The listing builds one solid part. Answer for the finished solid, in the listing's coordinates (mm). Face numbers are marked on the shaded views. A direction names the side the tool comes from. Give positions to 0.01 mm unless a question says otherwise; leave off trailing zeros. Loops run counter-clockwise (first coordinate to the right, second up) from the corner with the lowest first, then second, coordinate; pieces in that order, holes last. Notation, with made-up numbers: M 71,36 L 77,36 A29 ccw 77,73 Z; hole C -2,58.25 d5. An arc over 180 degrees is marked long. Return JSON: item names as keys, results as strings.
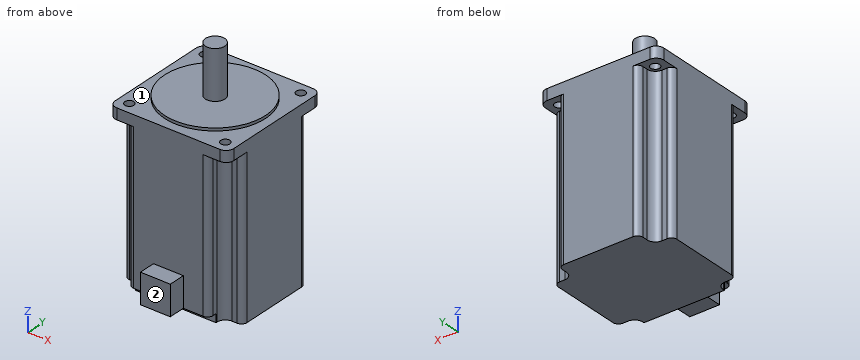
from build123d import *

# Parameters (mm, degrees)
SZKIC7_W                    = 21.6
SZKIC7_H                    = 21.6
DODANIE_WYCI_GNI_CIE5_DEPTH = 12
SZKIC8_W                    = 85.8
SZKIC8_H                    = 115
DODANIE_WYCI_GNI_CIE6_DEPTH = 85.8
SZKIC9_W                    = 85.8
SZKIC9_H                    = 78.988293657
DODANIE_WYCI_GNI_CIE7_DEPTH = 7
SZKIC10_W                   = 113
SZKIC10_H                   = 16.646355961
WYTNIJ_WYCI_GNI_CIE3_DEPTH  = 13.8
SZKIC11_W                   = 13.8
SZKIC11_H                   = 113
WYTNIJ_WYCI_GNI_CIE4_DEPTH  = 13.8
SZKIC12_W                   = 113
SZKIC12_H                   = 13.8
WYTNIJ_WYCI_GNI_CIE5_DEPTH  = 13.8
SZKIC13_W                   = 13.8
SZKIC13_H                   = 113
WYTNIJ_WYCI_GNI_CIE6_DEPTH  = 13.8
SZKIC14_R                   = 36.51
DODANIE_WYCI_GNI_CIE8_DEPTH = 2
OTW_R_POD_RUB_M121_D        = 14.05
OTW_R_POD_RUB_M121_DEPTH    = 2
SZKIC17_W                   = 7
SZKIC17_H                   = 37
OTW_R_6_6_6_6_1_D           = 6.6
OTW_R_6_6_6_6_1_DEPTH       = 45
ZAOKR_GLENIE1_R             = 4.000000016
ZAOKR_GLENIE2_R             = 5.6
ZAOKR_GLENIE3_R             = 5.99999999


with BuildPart() as part:
    # Szkic7 → Dodanie-wyciągnięcie5 (new body)
    with BuildSketch(Plane(origin=(0, -55, 0), x_dir=(-1, 0, 0), z_dir=(0, 1, 0))):
        with Locations((0, -104.2)):
            Rectangle(SZKIC7_W, SZKIC7_H)
    extrude(amount=DODANIE_WYCI_GNI_CIE5_DEPTH)

    # Szkic8 → Dodanie-wyciągnięcie6 (add)
    with BuildSketch(Plane(origin=(0, -43, 0), x_dir=(-1, 0, 0), z_dir=(0, 1, 0))):
        with Locations((0, -57.5)):
            Rectangle(SZKIC8_W, SZKIC8_H)
    extrude(amount=DODANIE_WYCI_GNI_CIE6_DEPTH)

    # Szkic9 → Dodanie-wyciągnięcie7 (add)
    with BuildSketch(Plane(origin=(0, 0, -121), x_dir=(-1, 0, 0), z_dir=(0, 0, -1))):
        with Locations((0, 3.305853172)):
            Rectangle(SZKIC9_W, SZKIC9_H)
    extrude(amount=-DODANIE_WYCI_GNI_CIE7_DEPTH)

    # Szkic10 → Wytnij-wyciągnięcie3 (cut)
    with BuildSketch(Plane.ZY.offset(42.9)):
        with Locations((-64.5, -37.423177981)):
            Rectangle(SZKIC10_W, SZKIC10_H)
    extrude(amount=-WYTNIJ_WYCI_GNI_CIE3_DEPTH, mode=Mode.SUBTRACT)

    # Szkic11 → Wytnij-wyciągnięcie4 (cut)
    with BuildSketch(Plane.XZ.offset(43)):
        with Locations((36, -64.5)):
            Rectangle(SZKIC11_W, SZKIC11_H)
    extrude(amount=-WYTNIJ_WYCI_GNI_CIE4_DEPTH, mode=Mode.SUBTRACT)

    # Szkic12 → Wytnij-wyciągnięcie5 (cut)
    with BuildSketch(Plane(origin=(42.9, 0, 0), x_dir=(0, 0, -1), z_dir=(1, 0, 0))):
        with Locations((64.5, 36)):
            Rectangle(SZKIC12_W, SZKIC12_H)
    extrude(amount=-WYTNIJ_WYCI_GNI_CIE5_DEPTH, mode=Mode.SUBTRACT)

    # Szkic13 → Wytnij-wyciągnięcie6 (cut)
    with BuildSketch(Plane(origin=(0, 42.8, 0), x_dir=(-1, 0, 0), z_dir=(0, 1, 0))):
        with Locations((36, -64.5)):
            Rectangle(SZKIC13_W, SZKIC13_H)
    extrude(amount=-WYTNIJ_WYCI_GNI_CIE6_DEPTH, mode=Mode.SUBTRACT)

    # Szkic14 → Dodanie-wyciągnięcie8 (add)
    with BuildSketch(Plane.XY):
        with Locations(Location((0, 0, 0), (0, 0, 90))):
            Circle(SZKIC14_R)
    extrude(amount=DODANIE_WYCI_GNI_CIE8_DEPTH)

    # Otwór pod śrubę M121
    with Locations(Plane.XY.offset(2)):
        with Locations((0, 0)):
            Hole(OTW_R_POD_RUB_M121_D / 2, depth=OTW_R_POD_RUB_M121_DEPTH)

    # Szkic17 → Obrót1 (revolve)
    with BuildSketch(Plane(origin=(0, 0, 0), x_dir=(1, 0, 0), z_dir=(0, 1, 0))):
        with Locations((3.5, -18.5)):
            Rectangle(SZKIC17_W, SZKIC17_H)
    revolve(axis=Axis((0, 0, 0), (0, 0, 1)))

    # Otwór Ø6.6 (6.6)1
    with Locations(Plane(origin=(0, 0, -8), x_dir=(-1, 0, 0), z_dir=(0, 0, -1))):
        with Locations((34.718942956, -34.718942956), (-34.718942956, -34.718942956), (-34.718942956, 34.718942956), (34.718942956, 34.718942956)):
            Hole(OTW_R_6_6_6_6_1_D / 2, depth=OTW_R_6_6_6_6_1_DEPTH)

    # Zaokrąglenie1
    zaokr_glenie1_edges = [part.edges().sort_by_distance(p)[0] for p in [
        (-42.9, 29, -64.5),
        (-29.1, 42.8, -64.5),
        (-29.1, -43, -61.5),
        (-42.9, -29.1, -64.5),
        (29.1, -43, -61.5),
        (42.9, -29.2, -64.5),
        (42.9, 29.1, -64.5),
        (29.1, 42.8, -64.5),
    ]]
    fillet(zaokr_glenie1_edges, radius=ZAOKR_GLENIE1_R)

    # Zaokrąglenie2
    zaokr_glenie2_edges = [part.edges().sort_by_distance(p)[0] for p in [
        (-42.9, 42.8, -4),
        (42.9, -43, -4),
        (42.9, 42.8, -4),
        (-42.9, -43, -4),
    ]]
    fillet(zaokr_glenie2_edges, radius=ZAOKR_GLENIE2_R)

    # Zaokrąglenie3
    zaokr_glenie3_edges = [part.edges().sort_by_distance(p)[0] for p in [
        (-29.1, 29, -64.5),
        (-29.1, -29.1, -64.5),
        (29.1, -29.2, -64.5),
        (29.1, 29.1, -64.5),
    ]]
    fillet(zaokr_glenie3_edges, radius=ZAOKR_GLENIE3_R)


solid = part.part
(1) Straight lines are drawn through the part: line 1 along Z through (x, y) = (6.5, 24); line 2 along Z through (x, y) = (33.5, 17); line 3 along Y through (x, z) = (-6.5, -70.5). For each, find the intervals that lie inside material, in ascending order.
Values follow:
{"line 1": "-121 to 2", "line 2": "-121 to 0", "line 3": "-43 to 42.8"}
(2) The part is cut by section A-A (y = 0). Determine the outline of the cut face in (x, z) (3 decimals), and give its area (3 significant figures).
Values follow:
{"outline": "M -42.9,-121 L 42.9,-121 L 42.9,0 L 36.51,0 L 36.51,2 L 7.025,2 L 7.025,0 L 7,0 L 7,37 L -7,37 L -7,0 L -7.025,0 L -7.025,2 L -36.51,2 L -36.51,0 L -42.9,0 Z", "area": "11,000 mm²"}
(3) The part is cut by section B-B (z = -19). Determine the outline of the cut face in (x, y), and give its area (3 significant figures).
Values follow:
{"outline": "M -42.9,-25.1 A4 ccw -38.9,-29.1 L -35.1,-29.1 A6 cw -29.1,-35.1 L -29.1,-39 A4 ccw -25.1,-43 L 25.1,-43 A4 ccw 29.1,-39 L 29.1,-35.2 A6 cw 35.1,-29.2 L 38.9,-29.2 A4 ccw 42.9,-25.2 L 42.9,25.1 A4 ccw 38.9,29.1 L 35.1,29.1 A6 cw 29.1,35.1 L 29.1,38.8 A4 ccw 25.1,42.8 L -25.1,42.8 A4 ccw -29.1,38.8 L -29.1,35 A6 cw -35.1,29 L -38.9,29 A4 ccw -42.9,25 Z", "area": "6,600 mm²"}
(4) The part is cut by section D-D (y = -20). Determine the outline of the cut face in (x, z), and give its area (3 significant figures).
Values follow:
{"outline": "M -42.9,-121 L 42.9,-121 L 42.9,0 L 30.54,0 L 30.54,2 L -30.54,2 L -30.54,0 L -42.9,0 Z", "area": "10,500 mm²"}
(5) The part is cut by section C-C (x = 0). Determine the outline of the cut face in (y, z) (3 decimals).
Values follow:
{"outline": "M -55,-115 L -36.188,-115 L -36.188,-121 L 42.8,-121 L 42.8,0 L 36.51,0 L 36.51,2 L 7.025,2 L 7.025,0 L 7,0 L 7,37 L -7,37 L -7,0 L -7.025,0 L -7.025,2 L -36.51,2 L -36.51,0 L -43,0 L -43,-93.4 L -55,-93.4 Z"}
(6) A tool of negligible diameter and unlimited length cuts with its end or side. For the marked faces 1 and 2, from which of +Z, -Z, +X, -X, +Y, -Y can it reach the whole face along a straight path? Write none if from no direction.
Values follow:
{"face 1": "+Z", "face 2": "+Z, -Z, +X, -X, -Y"}
(7) Given pin 1 (1.9 mm diameter, centred on y = 36, z = -70, fed in from -X); pin 2 (4 mm diameter, centred on x = 36.5, z = -87, fed in from -Y); pin 3 (1.9 mm diameter, centred on x = 37.5, z = -50.5, fed in from +Y), each flat-ended and moving along its own axis, determine where each tip first touches the part or whether it passes through.
Values follow:
{"pin 1": "x = -29.1", "pin 2": "y = -29.23", "pin 3": "y = 29.1"}
